from build123d import *

# Parameters (mm, degrees)
SKETCH1_W                = 58.3
SKETCH1_H                = 58.3
SKETCH1_W_2              = 28.3
SKETCH1_H_2              = 28.3
BOSS_EXTRUDE1_DEPTH      = 10
SKETCH4_W                = 60
SKETCH4_H                = 60
BOSS_EXTRUDE2_DEPTH      = 10
SKETCH6_W                = 60
SKETCH6_H                = 26.8
ESP32_DEPTH              = 6
SKETCH8_W                = 28.3
SKETCH8_H                = 28.3
CUT_EXTRUDE3_DEPTH       = 48
SKETCH10_W               = 30
SKETCH10_H               = 5
CUT_EXTRUDE5_DEPTH       = 50
CUT_EXTRUDE2_REACH       = 95.195
SKETCH7_W                = 50
SKETCH7_H                = 3.2
CUT_EXTRUDE6_START       = -10
CUT_EXTRUDE6_DEPTH       = 71.932070392
CUT_EXTRUDE7_START       = -25
CUT_EXTRUDE7_DEPTH       = 50
CUT_EXTRUDE8_REACH       = 102.747
SKETCH14_W               = 15
SKETCH14_H               = 3
CUT_EXTRUDE9_DEPTH       = 48
CHAMFER1_SIZE            = 7.5
CUT_EXTRUDE10_REACH      = 81.712
SKETCH15_R               = 2.65
SKETCH16_W               = 15.4
SKETCH16_H               = 16.6
CANBUS_DEPTH             = 3
SKETCH18_R               = 1.35
M2_CANBUS_HEAT_SET_DEPTH = 6
SKETCH19_R               = 2.75
CUT_EXTRUDE13_DEPTH      = 8
SKETCH20_R               = 2.75
CUT_EXTRUDE14_DEPTH      = 8
SKETCH21_R               = 2.75
CUT_EXTRUDE15_DEPTH      = 8
CUT_EXTRUDE16_START      = -8
SKETCH22_R               = 2.75
CUT_EXTRUDE16_DEPTH      = 8


# Read off the part's stored shape, not the designer's step: Cut-Extrude7
with BuildPart() as part:
    # Sketch1 → Boss-Extrude1 (new body)
    # profile 1 of 2: a face of its own
    with BuildSketch(Plane(origin=(0, 0, 0), x_dir=(1, 0, 0), z_dir=(0, 1, 0))):
        Rectangle(SKETCH1_W, SKETCH1_H)
        Rectangle(SKETCH1_W_2, SKETCH1_H_2, mode=Mode.SUBTRACT)
    # profile 2 of 2: a face of its own
    with BuildSketch(Plane(origin=(0, 0, 0), x_dir=(1, 0, 0), z_dir=(0, 1, 0))):
        Rectangle(SKETCH1_W_2, SKETCH1_H_2)
    extrude(amount=BOSS_EXTRUDE1_DEPTH)

    # Sketch2 → section 1 of loft1
    with BuildSketch(Plane(origin=(0, 40, 0), x_dir=(1, 0, 0), z_dir=(0, 1, 0)), mode=Mode.PRIVATE) as loft1_s1:
        with BuildLine():
            Line((-45, -45), (45, -45))
            Line((45, -45), (45, 45))
            Line((45, 45), (-45, 45))
            Line((-45, 45), (-45, -45))
        make_face()
    # loft from a face of the part (loft1)
    loft([part.faces().sort_by_distance((0, 10, 0))[0], loft1_s1.sketch])

    # Sketch4 → Boss-Extrude2 (add)
    with BuildSketch(Plane(origin=(0, 40, 0), x_dir=(1, 0, 0), z_dir=(0, 1, 0))):
        Rectangle(SKETCH4_W, SKETCH4_H)
    extrude(amount=BOSS_EXTRUDE2_DEPTH)

    # Sketch6 → ESP32 (cut)
    with BuildSketch(Plane(origin=(0, -9.857868483, -18.658426151), x_dir=(-1, 0, 0), z_dir=(0, -0.4671427704257183, -0.8841818998594039))):
        with Locations((0, 37.859030757)):
            Rectangle(SKETCH6_W, SKETCH6_H)
    extrude(amount=-ESP32_DEPTH, mode=Mode.SUBTRACT)

    # Sketch8 → Cut-Extrude3 (cut)
    with BuildSketch(Plane(origin=(0, 50, 0), x_dir=(1, 0, 0), z_dir=(0, 1, 0))):
        Rectangle(SKETCH8_W, SKETCH8_H)
    extrude(amount=-CUT_EXTRUDE3_DEPTH, mode=Mode.SUBTRACT)

    # Sketch10 → Cut-Extrude5 (cut)
    with BuildSketch(Plane(origin=(0, 0, 0), x_dir=(-1, 0, 0), z_dir=(0, -1, 0))):
        with Locations((0, 19.65)):
            Rectangle(SKETCH10_W, SKETCH10_H)
    extrude(amount=-CUT_EXTRUDE5_DEPTH, mode=Mode.SUBTRACT)

    # Cut-Extrude2: up to this plane
    cut_extrude2_end = Plane(origin=(-15, 50, -22.15), z_dir=(0, 0, -1))
    # Sketch7 → Cut-Extrude2 (cut, up to the surface)
    with BuildSketch(Plane(origin=(0, -7.055011861, -13.353334752), x_dir=(-1, 0, 0), z_dir=(0, -0.46714277042571845, -0.8841818998594037)), mode=Mode.PRIVATE) as cut_extrude2_sk1:
        with Locations((0, 47.659030757)):
            Rectangle(SKETCH7_W, SKETCH7_H)
    cut_extrude2_tool1 = split(extrude(cut_extrude2_sk1.sketch, amount=-CUT_EXTRUDE2_REACH, mode=Mode.PRIVATE), bisect_by=cut_extrude2_end, keep=Keep.BOTH, mode=Mode.PRIVATE)
    add(cut_extrude2_tool1.solids().sort_by_distance((0, 35.08424, -35.616906))[0], mode=Mode.SUBTRACT)
    # Sketch7 → Cut-Extrude2 (cut, up to the surface)
    with BuildSketch(Plane(origin=(0, -7.055011861, -13.353334752), x_dir=(-1, 0, 0), z_dir=(0, -0.46714277042571845, -0.8841818998594037)), mode=Mode.PRIVATE) as cut_extrude2_sk2:
        with Locations((0, 28.059030757)):
            Rectangle(SKETCH7_W, SKETCH7_H)
    cut_extrude2_tool2 = split(extrude(cut_extrude2_sk2.sketch, amount=-CUT_EXTRUDE2_REACH, mode=Mode.PRIVATE), bisect_by=cut_extrude2_end, keep=Keep.BOTH, mode=Mode.PRIVATE)
    add(cut_extrude2_tool2.solids().sort_by_distance((0, 17.754275, -26.460908))[0], mode=Mode.SUBTRACT)

    # Sketch11 → Cut-Extrude6 (cut, through all)
    with BuildSketch(Plane(origin=(0, 50, 0), x_dir=(1, 0, 0), z_dir=(0, 1, 0)).offset(CUT_EXTRUDE6_START)):
        Polygon((-25, 22.15), (25, 22.15), (15, 17.15), (-15, 17.15), align=None)
    extrude(amount=-CUT_EXTRUDE6_DEPTH, mode=Mode.SUBTRACT)

    # Cut-Extrude7 outline → Cut-Extrude7 (cut)
    with BuildSketch(Plane.YZ.offset(CUT_EXTRUDE7_START)):
        Polygon((40.38967366, -22.15), (21.841454111, -22.15), (21.504680154, -22.787427049), (36.005263311, -30.448568484), align=None)
    extrude(amount=CUT_EXTRUDE7_DEPTH, mode=Mode.SUBTRACT)

    # Cut-Extrude8: up to this plane
    cut_extrude8_end = Plane(origin=(18.658426151, -9.857868483, 0), z_dir=(-0.884181899859404, 0.4671427704257181, 0))
    # Sketch13 → Cut-Extrude8 (cut, up to the surface)
    with BuildSketch(Plane.ZY.offset(-30), mode=Mode.PRIVATE) as cut_extrude8_sk1:
        Polygon((-32.139713731, 15.658764159), (-40.548283598, 31.574038357), (-35.243192199, 34.376894979), (-26.834622332, 18.461620782), align=None)
    cut_extrude8_tool1 = split(extrude(cut_extrude8_sk1.sketch, amount=-CUT_EXTRUDE8_REACH, mode=Mode.PRIVATE), bisect_by=cut_extrude8_end, keep=Keep.BOTH, mode=Mode.PRIVATE)
    add(cut_extrude8_tool1.solids().sort_by_distance((30, 25.01783, -33.691453))[0], mode=Mode.SUBTRACT)

    # Sketch14 → Cut-Extrude9 (cut)
    with BuildSketch(Plane(origin=(0, 50, 0), x_dir=(1, 0, 0), z_dir=(0, 1, 0))):
        with Locations((0, 15.65)):
            Rectangle(SKETCH14_W, SKETCH14_H)
    extrude(amount=-CUT_EXTRUDE9_DEPTH, mode=Mode.SUBTRACT)

    # Chamfer1
    # the kernel refuses this chamfer: 7.5 mm, written as the material it adds along each edge
    with BuildSketch(Plane(origin=(15, 40, -17.15), x_dir=(-0.9996219169112968, 0, 0.02749587661058632), z_dir=(0, 1, 0))) as chamfer1_piece_1_section:
        Polygon((CHAMFER1_SIZE * 0.999621916911, -CHAMFER1_SIZE * 0.0274958766106), (-CHAMFER1_SIZE * 0.0274958766106, -CHAMFER1_SIZE * 0.999621916911), (0, 0), align=None)
    chamfer1_piece_1 = extrude(amount=10, mode=Mode.PRIVATE)
    chamfer1_piece_1 = split(chamfer1_piece_1, bisect_by=Plane(origin=(12.200765376, 42.822931518, -22.15), z_dir=(0, 0, 1)), keep=Keep.TOP, mode=Mode.PRIVATE)
    add(chamfer1_piece_1)
    with BuildSketch(Plane(origin=(-15, 40, -17.15), x_dir=(0.9996219169112968, 0, 0.02749587661058632), z_dir=(0, 1, 0))) as chamfer1_piece_2_section:
        Polygon((CHAMFER1_SIZE * 0.999621916911, CHAMFER1_SIZE * 0.0274958766106), (-CHAMFER1_SIZE * 0.0274958766106, CHAMFER1_SIZE * 0.999621916911), (0, 0), align=None)
    chamfer1_piece_2 = extrude(amount=10, mode=Mode.PRIVATE)
    chamfer1_piece_2 = split(chamfer1_piece_2, bisect_by=Plane(origin=(-12.200765376, 42.822931518, -22.15), z_dir=(0, 0, 1)), keep=Keep.TOP, mode=Mode.PRIVATE)
    add(chamfer1_piece_2)

    # Sketch15 → Cut-Extrude10 (cut, up to next)
    with BuildSketch(Plane(origin=(0, 2, 0), x_dir=(1, 0, 0), z_dir=(0, 1, 0)), mode=Mode.PRIVATE) as cut_extrude10_sk1:
        with Locations(Location((0, 0, 0), (0, 0, 270))):
            Circle(SKETCH15_R)
    cut_extrude10_tool1 = extrude(cut_extrude10_sk1.sketch, amount=-CUT_EXTRUDE10_REACH, mode=Mode.PRIVATE) & part.part
    add(cut_extrude10_tool1.solids().sort_by_distance((0, 2, 0))[0], mode=Mode.SUBTRACT)

    # Sketch16 → CANbus (cut)
    with BuildSketch(Plane(origin=(-18.658426151, -9.857868483, 0), x_dir=(0, 0, 1), z_dir=(-0.8841818998594037, -0.46714277042571845, 0))):
        with Locations((0, 40.759030757)):
            Rectangle(SKETCH16_W, SKETCH16_H)
    extrude(amount=-CANBUS_DEPTH, mode=Mode.SUBTRACT)

    # Sketch18 → M2-CANbus-Heat-Set (cut)
    with BuildSketch(Plane(origin=(-16.005880452, -8.456440172, 0), x_dir=(0, 0, 1), z_dir=(-0.8841818998594035, -0.46714277042571867, 0))):
        with Locations(Location((5.2, 45.898343703, 0), (0, 0, 270))):
            Circle(SKETCH18_R)
        with Locations(Location((5.2, 34.898343703, 0), (0, 0, 270))):
            Circle(SKETCH18_R)
    extrude(amount=-M2_CANBUS_HEAT_SET_DEPTH, mode=Mode.SUBTRACT)

    # Sketch19 → Cut-Extrude13 (cut)
    with BuildSketch(Plane(origin=(0, 0, -30), x_dir=(-1, 0, 0), z_dir=(0, 0, -1))):
        with Locations((-22.5, 45)):
            Circle(SKETCH19_R)
        with Locations((22.5, 45)):
            Circle(SKETCH19_R)
    extrude(amount=-CUT_EXTRUDE13_DEPTH, mode=Mode.SUBTRACT)

    # Sketch20 → Cut-Extrude14 (cut)
    with BuildSketch(Plane(origin=(30, 0, 0), x_dir=(0, 0, -1), z_dir=(1, 0, 0))):
        with Locations((0, 45)):
            Circle(SKETCH20_R)
    extrude(amount=-CUT_EXTRUDE14_DEPTH, mode=Mode.SUBTRACT)

    # Sketch21 → Cut-Extrude15 (cut)
    with BuildSketch(Plane.XY.offset(30)):
        with Locations((0, 45)):
            Circle(SKETCH21_R)
    extrude(amount=-CUT_EXTRUDE15_DEPTH, mode=Mode.SUBTRACT)

    # Sketch22 → Cut-Extrude16 (cut)
    with BuildSketch(Plane.ZY.offset(30).offset(CUT_EXTRUDE16_START)):
        with Locations(Location((0, 45, 0), (0, 0, 180))):
            Circle(SKETCH22_R)
    extrude(amount=CUT_EXTRUDE16_DEPTH, mode=Mode.SUBTRACT)


solid = part.part
The listing builds one solid part. Answer for the finished solid, in the listing's coordinates (mm). A direction names the side the tool comes from. Coordinates: 2 decimals unless noted, no trailing zeros.
1) Determine the mould class of faces 5 (the face through (-25.944, 42.273, 0.358)), 6 (the face through (10, 20, -17.15)), 7 (the face through (-14, 40, -20)) for opening direction Y: pulls with the +Y half, pulls with the -Y half, needs draft (parallel to the pull), parting line crosses it, or undercut.
2) Find section A-A on x = 0. Give the number of separate pieces and of enclosed holes in the cut face, then the cut area to 3 significant figures.
3) Find the intervals of material crossed by L1, parallel to X at y = 40.5, z = -11.5; L2, parallel to Z at x = 9.5, y = 3.5; L3, parallel to Y at x = -22, z = -24, in increasing order.
4) A tool of negligible diameter and unlimited length cuts with its end or side. For faces 1 (the face through (-22, 45, -22)), 2 (the face through (19, 42, -22.15)), 3 (the face through (-7.5, 26, -16)), 4 (the face through (0, 5, 29.15)), from which of +Z, -Z, +X, -X, +Y, -Y can it reach the whole face along a straight path? Write none if from no direction.
5) Flat-ended cylindrical pins translate along their axes: pin 1 Ø5 at (y, z) = (44.5, 3.5) entering from +X; pin 2 Ø3.5 at (x, y) = (-22.5, 45) entering from +Z; pin 3 Ø8 at (x, y) = (23.5, 5.5) entering from -Z. Find the tip coordinate at first contact, or state that the pin passes through.
Values:
1. face 5: undercut
1. face 6: needs draft
1. face 7: pulls with the -Y half
2. separate pieces: 5
2. enclosed holes: 0
2. area: 1,290 mm2
3. L1: x = -30 to -14.15, 14.15 to 30
3. L2: z = -29.15 to -22.15, -17.15 to -14.15, 14.15 to 29.15
3. L3: y = 0 to 17.24, 20.86 to 23.8, 47.7 to 50
4. face 1: -Z
4. face 2: none
4. face 3: +Y
4. face 4: +Z, +X, -X, -Y
5. pin 1: stops at x = 30
5. pin 2: stops at z = 30
5. pin 3: stops at z = -29.15
